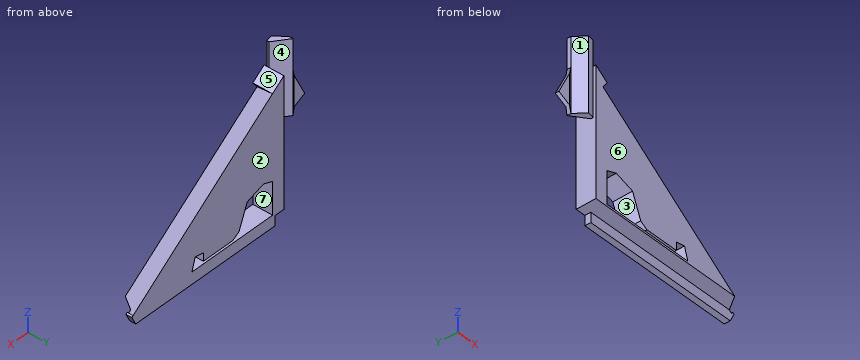
```python
from build123d import *

# Parameters (mm, degrees)
BOSS_EXTRUDE1_DEPTH = 25.4
SKETCH2_W           = 12.7
SKETCH2_H           = 17.78
CUT_EXTRUDE1_DEPTH  = 209.879612663
CUT_EXTRUDE2_DEPTH  = 95.896126628
CUT_EXTRUDE3_DEPTH  = 254


with BuildPart() as part:
    # Sketch1 → Boss-Extrude1 (new body)
    with BuildSketch(Plane(origin=(0, 0, 0), x_dir=(1, 0, 0), z_dir=(0, 1, 0))):
        Polygon((0, 0), (0, 101.6), (12.7, 101.6), (12.7, 114.3), (215.9, 114.3), (221.579612663, 102.940774674), (0, -63.146126628), (0, -94.896126628), (-19.05, -94.896126628), (-19.05, -56.796126628), (-41.768450651, -11.359225326), (-19.05, 0), align=None)
        Polygon((16.51, 99.016534905), (16.51, 57.380699548), (29.761390928, 52.687033829), (53.490710304, 60.611873008), (65.339387315, 90.173417518), (74.422473615, 95.748477248), (117.328122685, 95.748477248), (117.328122685, 85.363664607), (129.190216348, 83.158940906), (134.056716313, 99.016534905), align=None, mode=Mode.SUBTRACT)
    extrude(amount=BOSS_EXTRUDE1_DEPTH)

    # Sketch2 → Cut-Extrude1 (cut, through all)
    with BuildSketch(Plane.ZY.offset(-12.7)):
        with Locations((-107.95, 8.89)):
            Rectangle(SKETCH2_W, SKETCH2_H)
    extrude(amount=-CUT_EXTRUDE1_DEPTH, mode=Mode.SUBTRACT)

    # Sketch3 → Cut-Extrude2 (cut, through all)
    with BuildSketch(Plane(origin=(0, 0, 0), x_dir=(-1, 0, 0), z_dir=(0, 0, -1))):
        Polygon((26.279490994, 10.727129804), (19.05, 15.314148044), (19.05, 0), (41.768450651, 0), (41.768450651, 10.727129804), align=None)
        Polygon((8.25422712, 2.027835054), (0, 3.409743564), (0, 0), (19.05, 0), (19.05, 15.314148044), align=None)
        Polygon((19.05, 25.4), (0, 25.4), (0, 6.35), (19.05, 20.338025164), align=None)
        Polygon((41.768450651, 25.4), (19.05, 25.4), (19.05, 20.338025164), (26.279490994, 15.314148044), (41.768450651, 15.314148044), align=None)
    extrude(amount=-CUT_EXTRUDE2_DEPTH, mode=Mode.SUBTRACT)

    # Sketch4 → Cut-Extrude3 (cut)
    with BuildSketch(Plane(origin=(189.48572038, 0, -142.030648763), x_dir=(0, 1, 0), z_dir=(0.800169507, 0, -0.599773925))):
        Polygon((0, 40.087892142), (25.4, 50.527604994), (0, 50.527604994), align=None)
    extrude(amount=-CUT_EXTRUDE3_DEPTH, mode=Mode.SUBTRACT)


solid = part.part
```
CAD build for the part. Positions are in the model's coordinates, mm. Face numbers are marked on the shaded views. A direction names the side the tool comes from. Round coordinates to 2 decimals unless told otherwise and drop trailing zeros. Loops run counter-clockwise (first coordinate to the right, second up) from the corner with the lowest first, then second, coordinate; pieces in that order, holes last. Notation, with made-up numbers: (5, 32) - (25, 32) arc R24 cw to (25, 45) - close; hole circle Ø5 at (12.5, 26.25). An arc over 180 degrees is marked (long way). Return JSON: item names as keys, results as strings. Group by question number.
Q1. Band-saw the part on C-C on x = 78. Give the cut face in (y, z).
Q2. Band-saw the part on B-B on x = 206. Give the cut face in (y, z).
Q3. Band-saw the part on D-D on z = -22.5. Give the cut face in (x, y), plus the area to 3 significant figures.
Q4. Two-plate mould, pull along Z, no slides. Class the marked faces 5, 6 and 7: +Z half, -Z half, draft (parallel to the pull), parting line (faces both ways), or undercut.
Q5. Flat gauge pins, fed straight in: pin 1 Ø7.5 at (y, z) = (17.5, -68.5) entering from +X; pin 2 Ø3 at (y, z) = (5, 73.5) entering from +X; pin 3 Ø5 at (x, y) = (95, 10) entering from -Z; pin 4 Ø4 at (x, y) = (190, 17.5) entering from -Z. Where does each tip first touch, or does it go through?
Q6. Tool access for the marked faces 1, 2, 3 and 4: list every direction of +Z, -Z, +X, -X, +Y, -Y with a clear straight run to the whole face (end or side of a thin tool).
Q7. Band-saw the part on A-A on x = 20. Give the cut face in (y, z).
Q8. Drill centre lines: line 1 along X through (y, z) = (11.25, 37); line 2 along X through (y, z) = (3.75, -92.5); line 3 along Z through (x, y) = (8.5, 13.25). Where is each one in solid material? Low to high. Write a range as [from, to].
Solutions:
{
 "1": {"outline": "(0, -101.6) - (17.78, -101.6) - (17.78, -114.3) - (25.4, -114.3) - (25.4, -99.02) - (0, -99.02) - close; (0, -95.75) - (25.4, -95.75) - (25.4, 4.68) - (0, -8.37) - close"},
 "2": {"outline": "(5.28, -101.6) - (17.78, -101.6) - (17.78, -114.3) - (25.4, -114.3) - (25.4, -91.26) - close"},
 "3": {"outline": "(0, 0) - (96.86, 0) - (114.26, 25.4) - (0, 25.4) - close", "area": "2,680 mm^2"},
 "4": {"face 5": "+Z half", "face 6": "draft", "face 7": "undercut"},
 "5": {"pin 1": "stops at x = 175.84", "pin 2": "stops at x = 0", "pin 3": "stops at z = -101.6", "pin 4": "stops at z = -114.3"},
 "6": {"face 1": "+Z, -Z, -Y", "face 2": "+Z, -Z, +X, -X, +Y", "face 3": "+Y, -Y", "face 4": "+Z, -Z, +Y"},
 "7": {"outline": "(0, -101.6) - (17.78, -101.6) - (17.78, -114.3) - (25.4, -114.3) - (25.4, -99.02) - (0, -99.02) - close; (0, -56.14) - (25.4, -56.14) - (25.4, 48.15) - (0, 35.11) - close"},
 "8": {"line 1": "x = [-28.95, -25.46], [-15.75, -6.67], [0, 25.19]", "line 2": "x = [0, 16.51], [69.13, 117.33], [132.06, 192.81]", "line 3": "z = [-101.6, 56.77]"}
}
